Verification items for the finished model (mm, model axes). A direction names the side the tool comes from. Give positions to 0.01 mm unless a question says otherwise; leave off trailing zeros. Write each loop counter-clockwise with the first axis right and the second up, starting at its lowest first coordinate (ties: lowest second). Pieces come first, ordered by that corner, then holes. Notation, with made-up numbers: (62, 3) - (66, 3) arc R20 ccw to (66, 22) - close; hole circle Ø3 at (63, 67.5). An arc over 180 degrees is marked (long way). Put each result on its own line as item: value.
from build123d import *

# Parameters (mm, degrees)
F0_R     = 6.35
F1_DEPTH = 25.4


with BuildPart() as f1:
    # F0 (on Top) → F1 (new body)
    with BuildSketch(Plane.XY):
        with BuildLine():
            Line((1.27, 28.575), (0, 28.575))
            Line((0, 28.575), (-1.27, 28.575))
            Line((-1.27, 28.575), (-2.54, 24.982901))
            Line((-2.54, 24.982901), (-2.54, 23.072094))
            ThreePointArc((-2.54, 23.072094), (-2.991826, 21.728881), (-4.163596, 20.931809))
            ThreePointArc((-4.163596, 20.931809), (-5.551196, 21.219791), (-6.482654, 22.287851))
            Line((-6.482654, 22.287851), (-7.213888, 24.053207))
            Line((-7.213888, 24.053207), (-9.761852, 26.885866))
            Line((-9.761852, 26.885866), (-10.935179, 26.399858))
            Line((-10.935179, 26.399858), (-12.108506, 25.91385))
            Line((-12.108506, 25.91385), (-11.907196, 22.109175))
            Line((-11.907196, 22.109175), (-11.175962, 20.343819))
            ThreePointArc((-11.175962, 20.343819), (-11.07937, 18.929946), (-11.856917, 17.745131))
            ThreePointArc((-11.856917, 17.745131), (-13.249099, 17.48018), (-14.518383, 18.110485))
            Line((-14.518383, 18.110485), (-15.869528, 19.46163))
            Line((-15.869528, 19.46163), (-19.307551, 21.103602))
            Line((-19.307551, 21.103602), (-20.205576, 20.205576))
            Line((-20.205576, 20.205576), (-21.103602, 19.307551))
            Line((-21.103602, 19.307551), (-19.46163, 15.869528))
            Line((-19.46163, 15.869528), (-18.110485, 14.518383))
            ThreePointArc((-18.110485, 14.518383), (-17.48018, 13.249099), (-17.745131, 11.856917))
            ThreePointArc((-17.745131, 11.856917), (-18.929946, 11.07937), (-20.343819, 11.175962))
            Line((-20.343819, 11.175962), (-22.109175, 11.907196))
            Line((-22.109175, 11.907196), (-25.91385, 12.108506))
            Line((-25.91385, 12.108506), (-26.399858, 10.935179))
            Line((-26.399858, 10.935179), (-26.885866, 9.761852))
            Line((-26.885866, 9.761852), (-24.053207, 7.213888))
            Line((-24.053207, 7.213888), (-22.287851, 6.482654))
            ThreePointArc((-22.287851, 6.482654), (-21.219791, 5.551196), (-20.931809, 4.163596))
            ThreePointArc((-20.931809, 4.163596), (-21.728881, 2.991826), (-23.072094, 2.54))
            Line((-23.072094, 2.54), (-24.982901, 2.54))
            Line((-24.982901, 2.54), (-28.575, 1.27))
            Line((-28.575, 1.27), (-28.575, 0))
            Line((-28.575, 0), (-28.575, -1.27))
            Line((-28.575, -1.27), (-24.982901, -2.54))
            Line((-24.982901, -2.54), (-23.072094, -2.54))
            ThreePointArc((-23.072094, -2.54), (-21.728881, -2.991826), (-20.931809, -4.163596))
            ThreePointArc((-20.931809, -4.163596), (-21.219791, -5.551196), (-22.287851, -6.482654))
            Line((-22.287851, -6.482654), (-24.053207, -7.213888))
            Line((-24.053207, -7.213888), (-26.885866, -9.761852))
            Line((-26.885866, -9.761852), (-26.399858, -10.935179))
            Line((-26.399858, -10.935179), (-25.91385, -12.108506))
            Line((-25.91385, -12.108506), (-22.109175, -11.907196))
            Line((-22.109175, -11.907196), (-20.343819, -11.175962))
            ThreePointArc((-20.343819, -11.175962), (-18.929946, -11.07937), (-17.745131, -11.856917))
            ThreePointArc((-17.745131, -11.856917), (-17.48018, -13.249099), (-18.110485, -14.518383))
            Line((-18.110485, -14.518383), (-19.46163, -15.869528))
            Line((-19.46163, -15.869528), (-21.103602, -19.307551))
            Line((-21.103602, -19.307551), (-20.205576, -20.205576))
            Line((-20.205576, -20.205576), (-19.307551, -21.103602))
            Line((-19.307551, -21.103602), (-15.869528, -19.46163))
            Line((-15.869528, -19.46163), (-14.518383, -18.110485))
            ThreePointArc((-14.518383, -18.110485), (-13.249099, -17.48018), (-11.856917, -17.745131))
            ThreePointArc((-11.856917, -17.745131), (-11.07937, -18.929946), (-11.175962, -20.343819))
            Line((-11.175962, -20.343819), (-11.907196, -22.109175))
            Line((-11.907196, -22.109175), (-12.108506, -25.91385))
            Line((-12.108506, -25.91385), (-10.935179, -26.399858))
            Line((-10.935179, -26.399858), (-9.761852, -26.885866))
            Line((-9.761852, -26.885866), (-7.213888, -24.053207))
            Line((-7.213888, -24.053207), (-6.482654, -22.287851))
            ThreePointArc((-6.482654, -22.287851), (-5.551196, -21.219791), (-4.163596, -20.931809))
            ThreePointArc((-4.163596, -20.931809), (-2.991826, -21.728881), (-2.54, -23.072094))
            Line((-2.54, -23.072094), (-2.54, -24.982901))
            Line((-2.54, -24.982901), (-1.27, -28.575))
            Line((-1.27, -28.575), (0, -28.575))
            Line((0, -28.575), (1.27, -28.575))
            Line((1.27, -28.575), (2.54, -24.982901))
            Line((2.54, -24.982901), (2.54, -23.072094))
            ThreePointArc((2.54, -23.072094), (2.991826, -21.728881), (4.163596, -20.931809))
            ThreePointArc((4.163596, -20.931809), (5.551196, -21.219791), (6.482654, -22.287851))
            Line((6.482654, -22.287851), (7.213888, -24.053207))
            Line((7.213888, -24.053207), (9.761852, -26.885866))
            Line((9.761852, -26.885866), (10.935179, -26.399858))
            Line((10.935179, -26.399858), (12.108506, -25.91385))
            Line((12.108506, -25.91385), (11.907196, -22.109175))
            Line((11.907196, -22.109175), (11.175962, -20.343819))
            ThreePointArc((11.175962, -20.343819), (11.07937, -18.929946), (11.856917, -17.745131))
            ThreePointArc((11.856917, -17.745131), (13.249099, -17.48018), (14.518383, -18.110485))
            Line((14.518383, -18.110485), (15.869528, -19.46163))
            Line((15.869528, -19.46163), (19.307551, -21.103602))
            Line((19.307551, -21.103602), (20.205576, -20.205576))
            Line((20.205576, -20.205576), (21.103602, -19.307551))
            Line((21.103602, -19.307551), (19.46163, -15.869528))
            Line((19.46163, -15.869528), (18.110485, -14.518383))
            ThreePointArc((18.110485, -14.518383), (17.48018, -13.249099), (17.745131, -11.856917))
            ThreePointArc((17.745131, -11.856917), (18.929946, -11.07937), (20.343819, -11.175962))
            Line((20.343819, -11.175962), (22.109175, -11.907196))
            Line((22.109175, -11.907196), (25.91385, -12.108506))
            Line((25.91385, -12.108506), (26.399858, -10.935179))
            Line((26.399858, -10.935179), (26.885866, -9.761852))
            Line((26.885866, -9.761852), (24.053207, -7.213888))
            Line((24.053207, -7.213888), (22.287851, -6.482654))
            ThreePointArc((22.287851, -6.482654), (21.219791, -5.551196), (20.931809, -4.163596))
            ThreePointArc((20.931809, -4.163596), (21.728881, -2.991826), (23.072094, -2.54))
            Line((23.072094, -2.54), (24.982901, -2.54))
            Line((24.982901, -2.54), (28.575, -1.27))
            Line((28.575, -1.27), (28.575, 0))
            Line((28.575, 0), (28.575, 1.27))
            Line((28.575, 1.27), (24.982901, 2.54))
            Line((24.982901, 2.54), (23.072094, 2.54))
            ThreePointArc((23.072094, 2.54), (21.728881, 2.991826), (20.931809, 4.163596))
            ThreePointArc((20.931809, 4.163596), (21.219791, 5.551196), (22.287851, 6.482654))
            Line((22.287851, 6.482654), (24.053207, 7.213888))
            Line((24.053207, 7.213888), (26.885866, 9.761852))
            Line((26.885866, 9.761852), (26.399858, 10.935179))
            Line((26.399858, 10.935179), (25.91385, 12.108506))
            Line((25.91385, 12.108506), (22.109175, 11.907196))
            Line((22.109175, 11.907196), (20.343819, 11.175962))
            ThreePointArc((20.343819, 11.175962), (18.929946, 11.07937), (17.745131, 11.856917))
            ThreePointArc((17.745131, 11.856917), (17.48018, 13.249099), (18.110485, 14.518383))
            Line((18.110485, 14.518383), (19.46163, 15.869528))
            Line((19.46163, 15.869528), (21.103602, 19.307551))
            Line((21.103602, 19.307551), (20.205576, 20.205576))
            Line((20.205576, 20.205576), (19.307551, 21.103602))
            Line((19.307551, 21.103602), (15.869528, 19.46163))
            Line((15.869528, 19.46163), (14.518383, 18.110485))
            ThreePointArc((14.518383, 18.110485), (13.249099, 17.48018), (11.856917, 17.745131))
            ThreePointArc((11.856917, 17.745131), (11.07937, 18.929946), (11.175962, 20.343819))
            Line((11.175962, 20.343819), (11.907196, 22.109175))
            Line((11.907196, 22.109175), (12.108506, 25.91385))
            Line((12.108506, 25.91385), (10.935179, 26.399858))
            Line((10.935179, 26.399858), (9.761852, 26.885866))
            Line((9.761852, 26.885866), (7.213888, 24.053207))
            Line((7.213888, 24.053207), (6.482654, 22.287851))
            ThreePointArc((6.482654, 22.287851), (5.551196, 21.219791), (4.163596, 20.931809))
            ThreePointArc((4.163596, 20.931809), (2.991826, 21.728881), (2.54, 23.072094))
            Line((2.54, 23.072094), (2.54, 24.982901))
            Line((2.54, 24.982901), (1.27, 28.575))
        make_face()
        Circle(F0_R, mode=Mode.SUBTRACT)
    extrude(amount=F1_DEPTH)


solid = f1.part
Q1. Scan lines: line 1 along Y through (x, z) = (0, 19.5) (3 decimals); line 2 along X through (y, z) = (20.5, 8.5); line 3 along X through (y, z) = (19, 13.25). Record each from-to range of solid material in increasing order.
Answers follow:
line 1: y = -28.575 to -6.35, 6.35 to 28.575
line 2: x = -19.91 to -18.04, -11.24 to 11.24, 18.04 to 19.91
line 3: x = -20.96 to -15.41, -11.06 to 11.06, 15.41 to 20.96
Q2. Section check A-A, the plane y = 0. Record the cut outline in (x, z) (3 decimals).
Answers follow:
outline: (-28.575, 0) - (-6.35, 0) - (-6.35, 25.4) - (-28.575, 25.4) - close; (6.35, 0) - (28.575, 0) - (28.575, 25.4) - (6.35, 25.4) - close
Q3. Set-up check for faces 4 (the face through (11.074, -18.95, 12.522)), 5 (the face through (23.985, -12.006, 12.522)), 6 (the face through (-20.294, 17.613, 12.522)), 7 (the face through (21.713, -3.004, 12.522)), 8 (the face through (-15.184, 18.777, 12.522)): record each of +Z, -Z, +X, -X, +Y, -Y from which the full face is reachable in a straight line by a thin tool's end or side.
Answers follow:
face 4: +Z, -Z
face 5: +Z, -Z, -Y
face 6: +Z, -Z, -X
face 7: +Z, -Z, +X
face 8: +Z, -Z, +Y
Q4. Release check for a two-part mould opening along Y. For faces 1 (the face through (1.896, -26.804, 12.522)), 2 (the face through (-5.534, 21.21, 12.522)), 3 (the face through (-25.489, 8.506, 12.522)) record: released by +Y, released by -Y, zero draft, split by the parting line, or undercut.
Answers follow:
face 1: released by -Y
face 2: released by +Y
face 3: undercut
Q5. Go/stop test with flat-tipped pins: pin 1 Ø2 at (x, z) = (24.5, 13) entering from +Y; pin 2 Ø6 at (y, z) = (11.5, 6) entering from +X; pin 3 Ø1.5 at (y, z) = (24, 12) entering from -X. Record where each tip stops, or that it passes through.
Answers follow:
pin 1: stops at y = 12.09
pin 2: stops at x = 26.89
pin 3: stops at x = -12.05
